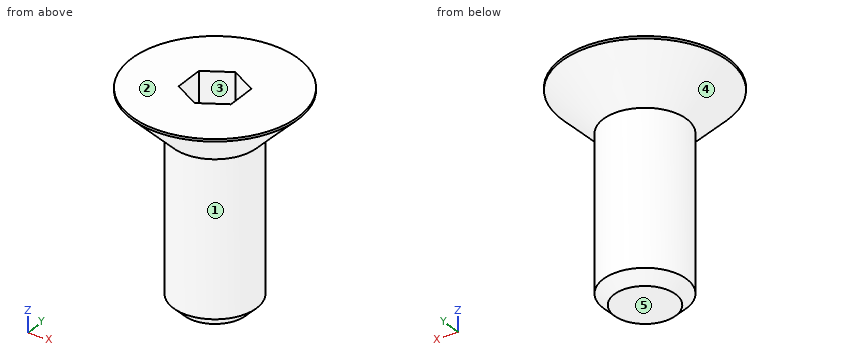
from build123d import *

# Parameters (mm, degrees)
CHAMFER1_SIZE      = 0.525
CUT_EXTRUDE2_DEPTH = 1.61


with BuildPart() as part:
    # Sketch1 → Revolve1 (revolve)
    with BuildSketch(Plane(origin=(0, 0, 0), x_dir=(0, 0, -1), z_dir=(1, 0, 0)), mode=Mode.PRIVATE) as revolve1_sk:
        Polygon((-2.7, 2), (5, 2), (5, 0), (-3.39, 0), (-3.39, 2), align=None)
    revolve(revolve1_sk.sketch.rotate(Axis((0, 0, 3.39), (0, 0, -1)), 180), axis=Axis((0, 0, 3.39), (0, 0, -1)))

    # Chamfer1
    chamfer1_edges = [part.edges().sort_by_distance(p)[0] for p in [
        (0, 2, -5),
    ]]
    chamfer(chamfer1_edges, length=CHAMFER1_SIZE)

    # Sketch7 → Revolve2 (revolve)
    with BuildSketch(Plane(origin=(0, 0, 0), x_dir=(0, 0, -1), z_dir=(1, 0, 0)), mode=Mode.PRIVATE) as revolve2_sk:
        Polygon((-5, 4), (-4.885, 4), (-2.7, 1.815), (-2.7, 0), (-5, 0), align=None)
    revolve(revolve2_sk.sketch.rotate(Axis((0, 0, 5), (0, 0, -1)), 180), axis=Axis((0, 0, 5), (0, 0, -1)))

    # Sketch5 → Cut-Extrude2 (cut)
    with BuildSketch(Plane.XY.offset(5)):
        Polygon((1.25, -0.721687836), (1.25, 0.721687836), (0, 1.443375673), (-1.25, 0.721687836), (-1.25, -0.721687836), (0, -1.443375673), align=None)
    extrude(amount=-CUT_EXTRUDE2_DEPTH, mode=Mode.SUBTRACT)


solid = part.part
Verification items for the finished model (mm, model axes). Face numbers are marked on the shaded views. A direction names the side the tool comes from. Give positions to 0.01 mm unless a question says otherwise; leave off trailing zeros. Loops run counter-clockwise (first coordinate to the right, second up) from the corner with the lowest first, then second, coordinate; pieces in that order, holes last.
1. Cross-section at B-B on y = 0. Record the cut outline in (x, z) (3 decimals).
Derived:
outline: (-4, 4.885) - (-2, 2.885) - (-2, -4.475) - (-1.475, -5) - (1.475, -5) - (2, -4.475) - (2, 2.885) - (4, 4.885) - (4, 5) - (1.25, 5) - (1.25, 3.39) - (-1.25, 3.39) - (-1.25, 5) - (-4, 5) - close
2. Cross-section at C-C on z = 2. Record the cut outline in (x, y), and give its area (3 significant figures).
Derived:
outline: circle Ø4 at (0, 0)
area: 12.6 mm2
3. Release check for a two-part mould opening along Y. For the marked faces 3, 4 and 5 record: +Y half, -Y half, draft (parallel to the pull), parting line (faces both ways), or undercut.
Derived:
face 3: undercut
face 4: parting line
face 5: draft
4. Go/stop test with flat-tipped pins: P1, Ø0.7, axis at y = 0, z = 4, coming from the +X side (3 decimals); P2, Ø2, axis at y = 2, z = -0.5, coming from the -X side; P3, Ø1.5, axis at y = 1, z = 2.5, coming from the -X side. Record where each tip stops, or that it passes through.
Derived:
P1: stops at x = 3.465
P2: stops at x = -1.73
P3: stops at x = -2.2
5. Tool access check on the marked faces 1 and 2. Record the directions out of +Z, -Z, +X, -X, +Y, -Y that give a thin tool (end or side, any length) a straight path to the whole face; none if there is none.
Derived:
face 1: -Z
face 2: +Z, +X, -X, +Y, -Y
6. Cross-section at A-A on z = 4. Record the cut outline in (x, y) (3 decimals).
Derived:
outline: circle Ø6.23 at (0, 0); hole (-1.25, -0.722) - (0, -1.443) - (1.25, -0.722) - (1.25, 0.722) - (0, 1.443) - (-1.25, 0.722) - close
7. Material ranges on probe 1 along Z at (x, y) = (-1, -0.25); probe 2 along Y at (x, z) = (2, 4.25); probe 3 along Y at (x, z) = (-0.25, -2.25), recorded low to high.
Derived:
probe 1: z = -5 to 3.39
probe 2: y = -2.71 to 2.71
probe 3: y = -1.98 to 1.98
